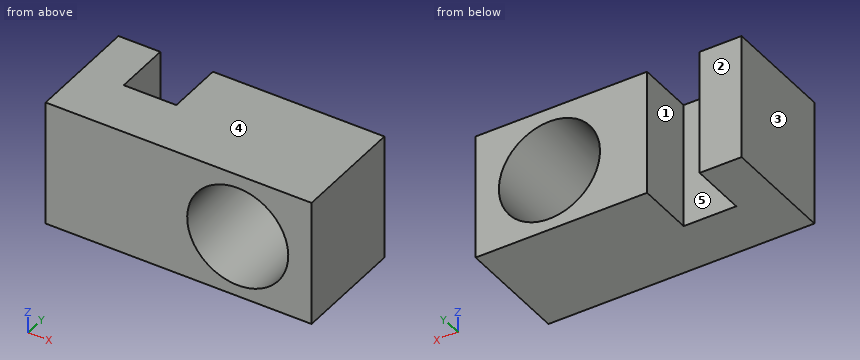
```python
from build123d import *

# Parameters (mm, degrees)
SKETCH1_W           = 42.285714286
SKETCH1_H           = 20
BOSS_EXTRUDE1_DEPTH = 18
SKETCH2_R           = 8.03891696
CUT_EXTRUDE1_DEPTH  = 18
SKETCH4_W           = 8.368646061
SKETCH4_H           = 9.041107824
CUT_EXTRUDE2_DEPTH  = 20


with BuildPart() as part:
    # Sketch1 → Boss-Extrude1 (new body)
    with BuildSketch(Plane(origin=(0, 0, 0), x_dir=(1, 0, 0), z_dir=(0, 1, 0))):
        with Locations((21.142857143, 10)):
            Rectangle(SKETCH1_W, SKETCH1_H)
    extrude(amount=BOSS_EXTRUDE1_DEPTH)

    # Sketch2 → Cut-Extrude1 (cut)
    with BuildSketch(Plane(origin=(0, 18, 0), x_dir=(1, 0, 0), z_dir=(0, 1, 0))):
        with Locations(Location((30.549434958, 10.165764801, 0), (0, 0, 270))):
            Circle(SKETCH2_R)
    extrude(amount=-CUT_EXTRUDE1_DEPTH, mode=Mode.SUBTRACT)

    # Sketch4 → Cut-Extrude2 (cut)
    with BuildSketch(Plane.XY):
        with Locations((10.8404183, 13.479446088)):
            Rectangle(SKETCH4_W, SKETCH4_H)
    extrude(amount=-CUT_EXTRUDE2_DEPTH, mode=Mode.SUBTRACT)


solid = part.part
```
Could you check a few things on this model? Use its own coordinates, in mm. Face numbers are marked on the shaded views. A direction names the side the tool comes from. Round coordinates to 2 decimals unless told otherwise and drop trailing zeros. Loops run counter-clockwise (first coordinate to the right, second up) from the corner with the lowest first, then second, coordinate; pieces in that order, holes last. Notation, with made-up numbers: (47, 46.5) - (70, 46.5) arc R10 cw to (70, 53.5) - close; hole circle Ø2 at (-39, 36.25). An arc over 180 degrees is marked (long way). Answer in a Markdown table with one row per item. Add a question column.
(1) I need wall thicknesses on line 1 along X through (y, z) = (2, -10); line 2 along X through (y, z) = (9, -8.5) (3 decimals); line 3 along X through (y, z) = (14.25, -6). Which ranges of each line are inside material? Lowest first, please.
(2) If we mould it in two halves opening along X, with no side actions, what happens to the marked faces 1, 2 and 3? For each: pulls with the +X half, pulls with the -X half, needs draft (parallel to the pull), parting line crosses it, or undercut.
(3) For the marked faces 4 and 5, which set-ups out of +Z, -Z, +X, -X, +Y, -Y let a thin tool reach every point of the face, with its end or its side?
(4) I'm going to push a flat-ended pin straight in: pin 1 (1.5 mm diameter, centred on x = 14, z = -6.5, fed in from +Y). Where does the tip first touch, or does it pass through?
(5) If we section it at C-C (y = 15): Please give me the cut outline in (x, z).
(6) If we section it at A-A (z = -12.75): Please give me the cut outline in (x, y).
(7) If we section it at B-B (x = 25): Please give me the cut outline in (y, z), plus the area to 3 significant figures.
(8) If we section it at D-D (z = -1.5): Please give me the cut outline in (x, y), plus the area to 3 significant figures.
Model answer:
| question | item | result |
|---|---|---|
| 1 | line 1 | x = 0 to 22.51, 38.59 to 42.29 |
| 1 | line 2 | x = 0 to 6.656, 15.025 to 22.685, 38.414 to 42.286 |
| 1 | line 3 | x = 0 to 6.66, 15.02 to 23.67, 37.42 to 42.29 |
| 2 | face 1 | undercut |
| 2 | face 2 | needs draft |
| 2 | face 3 | pulls with the -X half |
| 3 | face 4 | +Z, +X, -X, +Y, -Y |
| 3 | face 5 | +Z, -Z, +Y |
| 4 | pin 1 | stops at y = 8.96 |
| 5 | outline | (0, -20) - (6.66, -20) - (6.66, 0) - (0, 0) - close; (15.02, -20) - (42.29, -20) - (42.29, 0) - (15.02, 0) - close; hole circle Ø16.08 at (30.55, -10.17) |
| 6 | outline | (0, 0) - (22.94, 0) - (22.94, 18) - (15.02, 18) - (15.02, 8.96) - (6.66, 8.96) - (6.66, 18) - (0, 18) - close; (38.16, 0) - (42.29, 0) - (42.29, 18) - (38.16, 18) - close |
| 7 | outline | (0, -20) - (18, -20) - (18, -15.98) - (0, -15.98) - close; (0, -4.35) - (18, -4.35) - (18, 0) - (0, 0) - close |
| 7 | area | 151 mm² |
| 8 | outline | (0, 0) - (42.29, 0) - (42.29, 18) - (15.02, 18) - (15.02, 8.96) - (6.66, 8.96) - (6.66, 18) - (0, 18) - close |
| 8 | area | 685 mm² |
